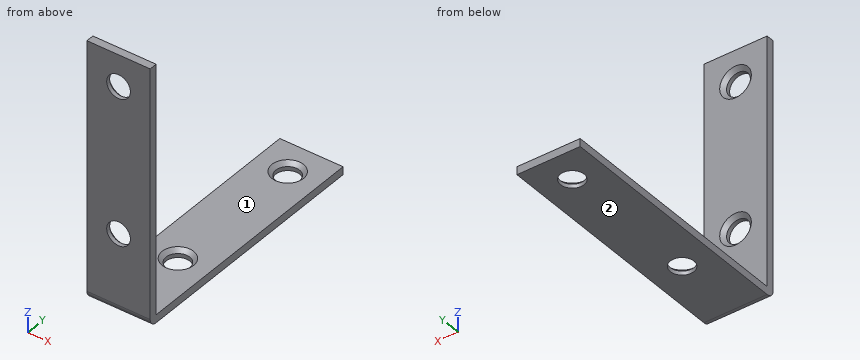
from build123d import *

# Parameters (mm, degrees)
F0_W     = 16
F0_H     = 65
F1_DEPTH = 2
F2_W     = 16
F2_H     = 2
F3_DEPTH = 63
F4_R     = 3
F5_DEPTH = 2.001
F6_R     = 3
F7_DEPTH = 65.001
F8_SIZE  = 1
F9_R     = 2


with BuildPart() as f1:
    # F0 (on Top) → F1 (new body)
    with BuildSketch(Plane.XY):
        with Locations((8, 32.5)):
            Rectangle(F0_W, F0_H)
    extrude(amount=F1_DEPTH)

    # F2 (on face) → F3 (join)
    with BuildSketch(Plane.XY.offset(2)):
        with Locations((8, 1)):
            Rectangle(F2_W, F2_H)
    extrude(amount=F3_DEPTH)

    # F4 (on face) → F5 (cut, through all)
    with BuildSketch(Plane.XY.offset(2)):
        with Locations((8, 57)):
            Circle(F4_R)
        with Locations((8, 20)):
            Circle(F4_R)
    extrude(amount=-F5_DEPTH, mode=Mode.SUBTRACT)

    # F6 (on face) → F7 (cut, through all)
    with BuildSketch(Plane.XZ):
        with Locations((8, 57)):
            Circle(F6_R)
        with Locations((8, 20)):
            Circle(F6_R)
    extrude(amount=-F7_DEPTH, mode=Mode.SUBTRACT)

    # F8
    f8_edges = [f1.edges().sort_by_distance(p)[0] for p in [
        (5, 2, 57),
        (5, 2, 20),
        (5, 20, 2),
        (5, 57, 2),
    ]]
    chamfer(f8_edges, length=F8_SIZE)

    # F9
    f9_edges = [f1.edges().sort_by_distance(p)[0] for p in [
        (8, 0, 0),
    ]]
    fillet(f9_edges, radius=F9_R)


solid = f1.part
Geometry check sheet. Reference: the model listing, model coordinates, mm. Face numbers are marked on the shaded views. A direction names the side the tool comes from. Give positions to 0.01 mm unless a question says otherwise; leave off trailing zeros. Loops run counter-clockwise (first coordinate to the right, second up) from the corner with the lowest first, then second, coordinate; pieces in that order, holes last. Notation, with made-up numbers: M 10,-2.75 L 19,-2.75 A20 cw 19,26.25 Z; hole C -11.5,-30.5 d7. An arc over 180 degrees is marked long. Answer as a JSON object with one key per item and string values. Group by question number.
Item 1: Sectioned sample at B-B on z = 20. Record the boundary of the cut face in (x, y), plus the area to 3 significant figures.
Item 2: Access from +Z, -Z, +X, -X, +Y, -Y to the whole of each face (thin tool, end or side, straight path). Record for the marked faces 1 and 2.
Item 3: Gauge pin test, flat ends, axial feed: pin 1 (3 mm diameter, centred on x = 3, z = 13.5, fed in from +Y); pin 2 (5 mm diameter, centred on x = 8, z = 57, fed in from +Y); pin 3 (4 mm diameter, centred on x = 6.5, y = 49, fed in from +Z). Record the tip position at first contact, or that the pin passes through.
Item 4: Sectioned sample at A-A on x = 8. Give the number of separate pieces and of enclosed holes in the cut face, plus the area to 3 significant figures.
Item 5: Sectioned sample at D-D on x = 1. Record the boundary of the cut face in (y, z), plus the area to 3 significant figures.
Item 6: Material ranges on L1, parallel to Y at x = 8, z = 0.45; L2, parallel to Z at x = 8, y = 0.35; L3, parallel to Z at x = 8, y = 0.25, recorded low to high.
Findings below:
{
 "1": {"outline": "M 0,0 L 5,0 L 5,1 L 4,2 L 0,2 Z; M 11,0 L 16,0 L 16,2 L 12,2 L 11,1 Z", "area": "19.0 mm2"},
 "2": {"face 1": "+Z, +X, -X, +Y", "face 2": "-Z, +X, -X, +Y, -Y"},
 "3": {"pin 1": "y = 2", "pin 2": "through", "pin 3": "z = 2"},
 "4": {"separate pieces": "5", "enclosed holes": "0", "area": "203 mm2"},
 "5": {"outline": "M 0,2 A2 ccw 2,0 L 65,0 L 65,2 L 2,2 L 2,65 L 0,65 Z", "area": "255 mm2"},
 "6": {"L1": "0.74 to 17, 23 to 54, 60 to 65", "L2": "0.87 to 17, 23 to 54, 60 to 65", "L3": "1.03 to 17, 23 to 54, 60 to 65"}
}
